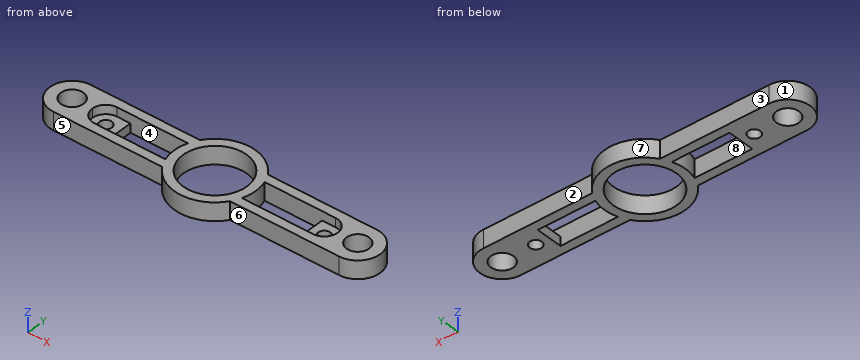
```python
from build123d import *

# Parameters (mm, degrees)
F0_R     = 4
F0_R_2   = 11.2530001
F1_DEPTH = 6.35
F2_R     = 2.15265
F3_DEPTH = 6.35
F4_W     = 9.525
F4_H     = 9.525
F5_DEPTH = 3.175
F6_R     = 4.76249


# Not quite as in the source:
# - a fillet or chamfer is up to 0.001 mm smaller than in the source, because OpenCascade refuses the exact size


with BuildPart() as f1:
    # F0 (on Top) → F1 (new body)
    with BuildSketch(Plane.XY):
        with BuildLine():
            Line((-12.0483725306, 7.9375), (-50.8, 7.9375))
            ThreePointArc((-50.8, 7.9375), (-58.7375, 0), (-50.8, -7.9375))
            Line((-50.8, -7.9375), (-12.0483725306, -7.9375))
            ThreePointArc((-12.0483725306, -7.9375), (0, -14.4280001), (12.0483725306, -7.9375))
            Line((12.0483725306, -7.9375), (50.8, -7.9375))
            ThreePointArc((50.8, -7.9375), (58.7375, 0), (50.8, 7.9375))
            Line((50.8, 7.9375), (12.0483725306, 7.9375))
            ThreePointArc((12.0483725306, 7.9375), (0, 14.4280001), (-12.0483725306, 7.9375))
        make_face()
        with Locations((-50.8, 0)):
            Circle(F0_R, mode=Mode.SUBTRACT)
        Circle(F0_R_2, mode=Mode.SUBTRACT)
        with Locations((50.8, 0)):
            Circle(F0_R, mode=Mode.SUBTRACT)
    extrude(amount=F1_DEPTH)

    # F2 (on face) → F3 (cut, through all)
    with BuildSketch(Plane.XY.offset(6.35)):
        with BuildLine():
            ThreePointArc((-13.6193164526, -4.7625), (-14.4280001, 0), (-13.6193164526, 4.7625))
            Line((-13.6193164526, 4.7625), (-34.1, 4.7625))
            Line((-34.1, 4.7625), (-34.1, -4.7625))
            Line((-34.1, -4.7625), (-13.6193164526, -4.7625))
        make_face()
        with BuildLine():
            Line((34.1, 4.7625), (13.6193164526, 4.7625))
            ThreePointArc((13.6193164526, 4.7625), (14.4280001, 0), (13.6193164526, -4.7625))
            Line((13.6193164526, -4.7625), (34.1, -4.7625))
            Line((34.1, -4.7625), (34.1, 4.7625))
        make_face()
        with Locations((-38.8625, 0)):
            Circle(F2_R)
        with Locations((38.8625, 0)):
            Circle(F2_R)
    extrude(amount=-F3_DEPTH, mode=Mode.SUBTRACT)

    # F4 (on face) → F5 (cut)
    with BuildSketch(Plane.XY.offset(6.35)):
        with Locations((-38.8625, 0)):
            Rectangle(F4_W, F4_H)
        with Locations((38.8625, 0)):
            Rectangle(F4_W, F4_H)
    extrude(amount=-F5_DEPTH, mode=Mode.SUBTRACT)

    # F6 (radius 4.7625 in the source; OpenCascade refuses exactly that, so slightly less here)
    f6_edges = [f1.edges().sort_by_distance(p)[0] for p in [
        (-43.625, 4.7625, 4.7625),
        (-43.625, -4.7625, 4.7625),
        (43.625, 4.7625, 4.7625),
        (43.625, -4.7625, 4.7625),
    ]]
    fillet(f6_edges, radius=F6_R)


solid = f1.part
```
Geometry check sheet. Reference: the model listing, model coordinates, mm. Face numbers are marked on the shaded views. A direction names the side the tool comes from. Round coordinates to 2 decimals unless told otherwise and drop trailing zeros. Write each loop counter-clockwise with the first axis right and the second up, starting at its lowest first coordinate (ties: lowest second). Pieces come first, ordered by that corner, then holes. Notation, with made-up numbers: (8, 43.25) -> (40, 43.25) arc R25 ccw to (40, 81.25) -> close; hole circle Ø3 at (72.25, 54.5). An arc over 180 degrees is marked (long way). Put each result on its own line as item: value.
1) Cross-section at B-B, the plane z = 4.5. Give the number of separate pieces and of enclosed holes in the cut face, plus the area to 3 significant figures.
Recorded:
separate pieces: 1
enclosed holes: 5
area: 991 mm2
2) Cross-section at C-C, the plane x = 0. Enter the section's corners in (y, z).
Recorded:
outline: (-14.43, 0) -> (-11.25, 0) -> (-11.25, 6.35) -> (-14.43, 6.35) -> close; (11.25, 0) -> (14.43, 0) -> (14.43, 6.35) -> (11.25, 6.35) -> close
3) Release check for a two-part mould opening along X. For the marked faces 6, 7 and 8 record: pulls with the +X half, pulls with the -X half, needs draft (parallel to the pull), parting line crosses it, or undercut.
Recorded:
face 6: needs draft
face 7: parting line crosses it
face 8: undercut
4) Access from +Z, -Z, +X, -X, +Y, -Y to the whole of each face (thin tool, end or side, straight path). Record for the marked faces 1, 2, 3, 4 and 5.
Recorded:
face 1: +Z, -Z, -X
face 2: +Z, -Z, +X, +Y
face 3: +Z, -Z, -X, +Y
face 4: +Z
face 5: +Z, -Z, -X, -Y
5) Cross-section at A-A, the plane x = -30. Enter the section's corners in (y, z), plus the area to 3 significant figures.
Recorded:
outline: (-7.94, 0) -> (-4.76, 0) -> (-4.76, 6.35) -> (-7.94, 6.35) -> close; (4.76, 0) -> (7.94, 0) -> (7.94, 6.35) -> (4.76, 6.35) -> close
area: 40.3 mm2
6) Cross-section at D-D, the plane y = 12.25. Enter the section's corners in (x, z), plus the area to 3 significant figures.
Recorded:
outline: (-7.62, 0) -> (7.62, 0) -> (7.62, 6.35) -> (-7.62, 6.35) -> close
area: 96.8 mm2
7) Thickness scan on probe 1 along Y at (x, z) = (28, 1); probe 2 along Y at (x, z) = (50.8, 5); probe 3 along X at (y, z) = (2.25, 3.75). Record the ranges inside material, lowest first. Write a range as from..to.
Recorded:
probe 1: y = -7.94..-4.76, 4.76..7.94
probe 2: y = -7.94..-4, 4..7.94
probe 3: x = -58.41..-54.11, -47.49..-43.06, -14.25..-11.03, 11.03..14.25, 43.06..47.49, 54.11..58.41
8) Depth check by flat-ended pin: P1, Ø9, axis at x = 50.8, y = 0, coming from the -Z side; P2, Ø1.9, axis at x = -31, z = 3.5, coming from the -Y side; P3, Ø2, axis at x = -10.5, z = 2, coming from the +Y side; P4, Ø2, axis at y = -11, z = 5.5, coming from the +X side. Enter the tip coordinate at first touch or a pass-through.
Recorded:
P1: stops at z = 0
P2: stops at y = -7.94
P3: stops at y = 10.86
P4: stops at x = 10.4
